Drawing for the job (mm, zero at the part's lowest x, y, z). Round coordinates to 2 decimals unless told otherwise and drop trailing zeros. Write each loop counter-clockwise with the first axis right and the second up, starting at its lowest first coordinate (ties: lowest second). Pieces come first, ordered by that corner, then holes. Notation, with made-up numbers: M -35,41.25 L 20,41.25 A14 cw 20,50.25 Z; hole C 71.5,-16.75 d4. An arc over 180 degrees is marked long. Use a Markdown table: item, result. Add a question column.
1) Two-plate mould, pull along Z, no slides. Class the marked faces 1 and 2: released by +Z, released by -Z, zero draft, split by the parting line, or undercut.
2) Wall check: probe 1 along X at (y, z) = (7.75, 78.5); probe 2 along Z at (x, y) = (172, 10.75); probe 3 along X at (y, z) = (4.75, 66). Give the ranges that are in metal, low to high.
3) Slice it at A-A on y = 10.5. Write the cut outline in (x, z), plus the area to 3 significant figures.
4) Slice it at B-B on z = 42. Write the cut outline in (x, y).
5) Drop flat-ended pins along their axis: P1, Ø2, axis at x = 95, y = 10.5, coming from the -Z side; P2, Ø10, axis at x = 28, z = 70, coming from the +Y side; P3, Ø4.5, axis at y = 10.5, z = 45, coming from the -X side. Give the stop position or say it passes through.
6) Slice it at C-C on x = 57. Write the cut outline in (y, z), plus the area to 3 significant figures.
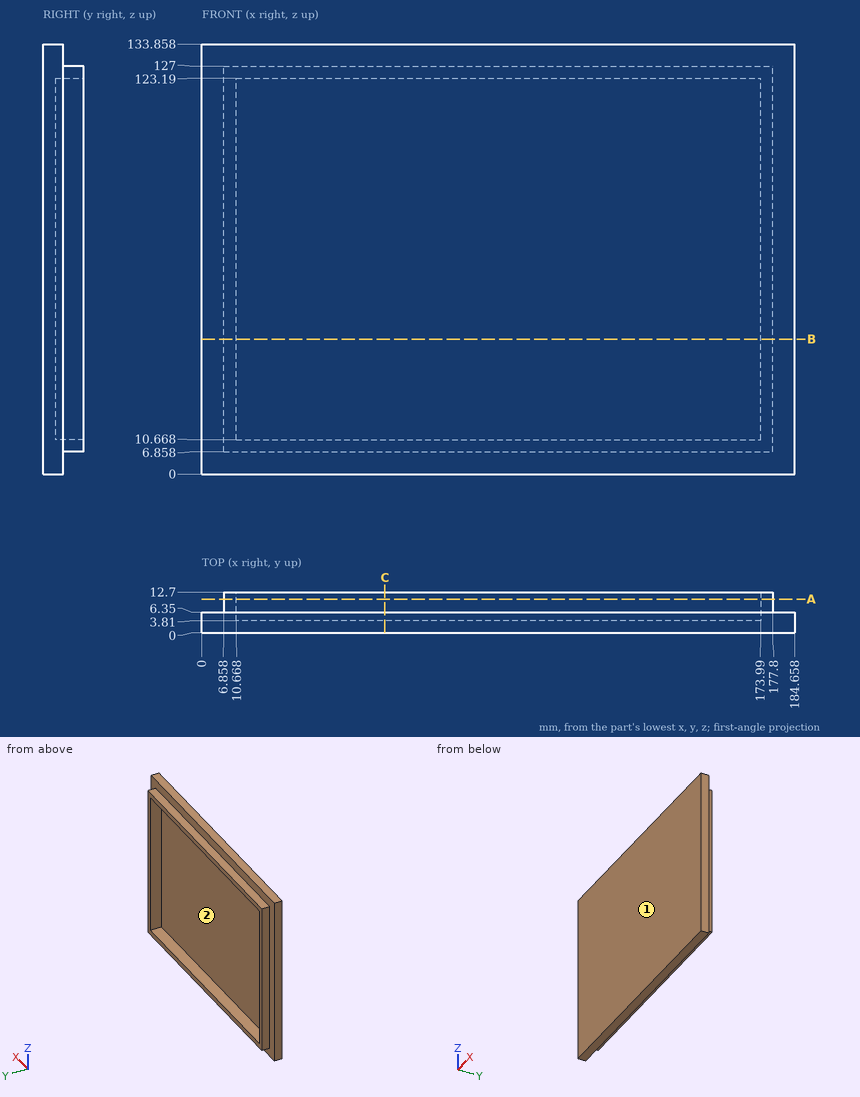
Entries:
| question | item | result |
|---|---|---|
| 1 | face 1 | zero draft |
| 1 | face 2 | undercut |
| 2 | probe 1 | x = 6.86 to 10.67, 173.99 to 177.8 |
| 2 | probe 2 | z = 6.86 to 10.67, 123.19 to 127 |
| 2 | probe 3 | x = 0 to 10.67, 173.99 to 184.66 |
| 3 | outline | M 6.86,6.86 L 177.8,6.86 L 177.8,127 L 6.86,127 Z; hole M 10.67,10.67 L 173.99,10.67 L 173.99,123.19 L 10.67,123.19 Z |
| 3 | area | 2,160 mm^2 |
| 4 | outline | M 0,0 L 184.66,0 L 184.66,6.35 L 177.8,6.35 L 177.8,12.7 L 173.99,12.7 L 173.99,3.81 L 10.67,3.81 L 10.67,12.7 L 6.86,12.7 L 6.86,6.35 L 0,6.35 Z |
| 5 | P1 | stops at z = 6.86 |
| 5 | P2 | stops at y = 3.81 |
| 5 | P3 | stops at x = 6.86 |
| 6 | outline | M 0,0 L 6.35,0 L 6.35,6.86 L 12.7,6.86 L 12.7,10.67 L 3.81,10.67 L 3.81,123.19 L 12.7,123.19 L 12.7,127 L 6.35,127 L 6.35,133.86 L 0,133.86 Z |
| 6 | area | 613 mm^2 |
